For this review, take the finished solid that the model builds, in its own axes (mm). Round coordinates to 2 decimals unless told otherwise and drop trailing zeros. Write each loop counter-clockwise with the first axis right and the second up, starting at its lowest first coordinate (ties: lowest second). Pieces come first, ordered by that corner, then holes. Notation, with made-up numbers: (81, -28.5) -> (140, -28.5) arc R7 cw to (140, -19.5) -> close; hole circle Ø7 at (58, 75.5). An arc over 180 degrees is marked (long way). Write each question's results on one line, items separated by ' | '. Start each with the question number.
Item 1: Add section B-B (y = 18). State the section outline as (x, z) points, plus the area to 3 significant figures.
Item 2: Clearance check with a flat-ended pin moving along its axis: pin 1 (8 mm diameter, centred on y = 31, z = -616, fed in from +X). State where the tip first meets the part, or that it passes through.
Item 3: Add section A-A (z = -382.5). State the section outline as (x, y) points.
Item 4: To check wall thickness, follow line 1 along Y through (x, z) = (-1, -812.5); line 2 along X through (y, z) = (3, -723.5); line 3 along X through (y, z) = (19.5, -654.5). State the ranges of each line that lie inside material, in increasing order.
from build123d import *

# Parameters (mm, degrees)
BODY_DEPTH                      = 885
SCHNITT_LINEAR_AUSTRAGEN2_DEPTH = 885


with BuildPart() as part:
    # Model → Body (new body)
    with BuildSketch(Plane.XY):
        with BuildLine():
            Line((1.878084628, 39.104629182), (2.149753631, 39.265339178))
            ThreePointArc((2.149753631, 39.265339178), (1.179756728, 40.293308137), (0.151359725, 39.323765061))
            Line((0.151359725, 39.323765061), (0.072230593, 36.617684207))
            ThreePointArc((0.072230593, 36.617684207), (0.185489498, 36.248958877), (0.499809768, 36.025377312))
            Line((0.499809768, 36.025377312), (1.261518581, 35.79721719))
            ThreePointArc((1.261518581, 35.79721719), (2.002767255, 35.193636824), (2.100773109, 34.24276685))
            ThreePointArc((2.100773109, 34.24276685), (0.243973004, 18.756791477), (3.6673456, 3.540232734))
            ThreePointArc((3.6673456, 3.540232734), (3.762278433, 3.217871116), (3.78778584, 2.882791084))
            Line((3.78778584, 2.882791084), (3.698637797, -0.165904914))
            ThreePointArc((3.698637797, -0.165904914), (3.256166133, -1.000710488), (2.324510635, -1.157871399))
            Line((2.324510635, -1.157871399), (2.175621232, -1.113273313))
            ThreePointArc((2.175621232, -1.113273313), (1.997498531, -0.968129525), (1.974178859, -0.739545604))
            Line((1.974178859, -0.739545604), (0.400869285, -0.26828127))
            Line((0.400869285, -0.26828127), (-0.708129005, -0.492759369))
            ThreePointArc((-0.708129005, -0.492759369), (-1.196616048, -1.010909594), (-1.76840947, -0.586466985))
            ThreePointArc((-1.76840947, -0.586466985), (-3.655039198, 17.174334722), (-1.986171677, 34.956919747))
            ThreePointArc((-1.986171677, 34.956919747), (-1.847587365, 35.23826116), (-1.585988155, 35.411248024))
            Line((-1.585988155, 35.411248024), (-1.044699422, 35.590524224))
            ThreePointArc((-1.044699422, 35.590524224), (-0.684484453, 35.850559404), (-0.538564027, 36.270178693))
            Line((-0.538564027, 36.270178693), (-0.448759368, 39.341314215))
            ThreePointArc((-0.448759368, 39.341314215), (1.197302045, 40.893129938), (2.749873366, 39.247781189))
            ThreePointArc((2.749873366, 39.247781189), (2.372981432, 38.816883238), (1.878084628, 39.104629182))
        make_face()
    extrude(amount=-BODY_DEPTH)

    # Skizze3 → Schnitt-Linear austragen2 (cut)
    with BuildSketch(Plane.XY):
        with BuildLine():
            Line((-0.588130108, 3.611006063), (-0.708129005, -0.492759369))
            Line((-0.708129005, -0.492759369), (0.400869714, -0.268279835))
            Line((0.400869714, -0.268279835), (1.974178926, -0.739545381))
            ThreePointArc((1.974178926, -0.739545381), (2.119322659, -0.561422774), (2.347906465, -0.53810304))
            Line((2.347906465, -0.53810304), (2.496795914, -0.582700974))
            ThreePointArc((2.496795914, -0.582700974), (2.904733153, -0.513885986), (3.0984751, -0.148355754))
            Line((3.0984751, -0.148355754), (3.128422919, 0.875806051))
            ThreePointArc((3.128422919, 0.875806051), (2.924721832, 2.674341696), (2.225195598, 4.343739086))
            ThreePointArc((2.225195598, 4.343739086), (0.543823558, 5.032117471), (-0.588130108, 3.611006063))
        make_face()
    extrude(amount=-SCHNITT_LINEAR_AUSTRAGEN2_DEPTH, mode=Mode.SUBTRACT)


with BuildPart() as schnitt_linear_austragen2_kept_piece:
    # of the separate pieces the step leaves, the one the design keeps (schnitt_linear_austragen2_pieces_kept)
    add(part.part.solids().sort_by_distance((-1.986171677, 34.956919747, 0))[0])


solid = schnitt_linear_austragen2_kept_piece.part
Responses:
1) outline: (-3.66, -885) -> (0.29, -885) -> (0.29, 0) -> (-3.66, 0) -> close | area: 3,490 mm^2
2) pin 1: stops at x = 2.15
3) outline: (-1.99, 34.96) arc R89.72 ccw to (-1.77, -0.59) arc R0.54 ccw to (-0.71, -0.49) -> (-0.59, 3.61) arc R1.51 cw to (2.23, 4.34) arc R6.39 cw to (3.13, 0.88) -> (3.1, -0.15) arc R0.47 cw to (2.5, -0.58) -> (2.35, -0.54) arc R0.3 ccw to (2.18, -1.11) -> (2.32, -1.16) arc R1.07 ccw to (3.7, -0.17) -> (3.79, 2.88) arc R1.6 ccw to (3.67, 3.54) arc R46.01 cw to (2.1, 34.24) arc R1.25 ccw to (1.26, 35.8) -> (0.5, 36.03) arc R0.6 cw to (0.07, 36.62) -> (0.15, 39.32) arc R1 cw to (2.15, 39.27) -> (1.88, 39.1) arc R0.45 ccw to (2.75, 39.25) arc R1.6 ccw to (-0.45, 39.34) -> (-0.54, 36.27) arc R0.74 cw to (-1.04, 35.59) -> (-1.59, 35.41) arc R0.6 ccw to start
4) line 1: y = -0.95 to 35.61 | line 2: x = -2.44 to -0.61, 2.83 to 3.79 | line 3: x = -3.64 to 0.21
